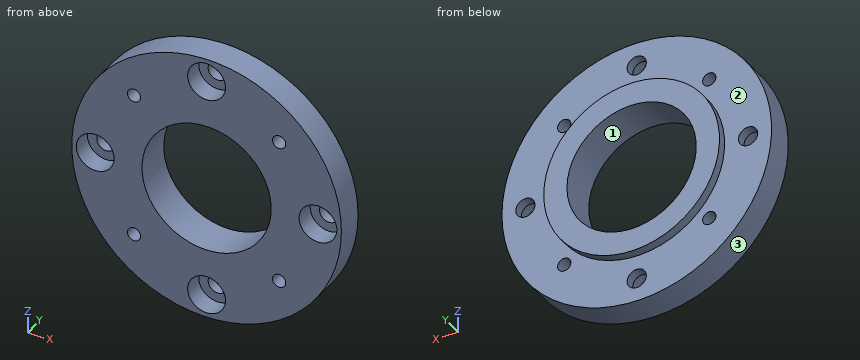
from build123d import *

# Parameters (mm, degrees)
SKETCH2_R                                      = 22.985
SKETCH2_R_2                                    = 1.63
SKETCH2_R_3                                    = 1.13
SKETCH2_R_4                                    = 14.985
SKETCH2_R_5                                    = 11.025
BOSS_EXTRUDE1_DEPTH                            = 4.95
BOSS_EXTRUDE2_START                            = 4.95
SKETCH2_3_R                                    = 14.985
SKETCH2_3_R_2                                  = 11.025
BOSS_EXTRUDE2_DEPTH                            = 1.52
F_4_40_TAPPED_HOLE1_D                          = 2.2606
CBORE_FOR_4_SOCKET_HEAD_CAP_SCREW1_D           = 3.2639
CBORE_FOR_4_SOCKET_HEAD_CAP_SCREW1_CBORE_D     = 6.450000054
CBORE_FOR_4_SOCKET_HEAD_CAP_SCREW1_CBORE_DEPTH = 3.300000004


with BuildPart() as part:
    # Sketch2 → Boss-Extrude1 (new body)
    with BuildSketch(Plane(origin=(0, 0, 0), x_dir=(1, 0, 0), z_dir=(0, 1, 0))):
        Circle(SKETCH2_R)
        with Locations((-18.99, 0)):
            Circle(SKETCH2_R_2, mode=Mode.SUBTRACT)
        with Locations((0, -18.99)):
            Circle(SKETCH2_R_2, mode=Mode.SUBTRACT)
        with Locations((18.99, 0)):
            Circle(SKETCH2_R_2, mode=Mode.SUBTRACT)
        with Locations((0, 18.99)):
            Circle(SKETCH2_R_2, mode=Mode.SUBTRACT)
        with Locations((12.367297603, -12.367297603)):
            Circle(SKETCH2_R_3, mode=Mode.SUBTRACT)
        with Locations((-12.367297603, -12.367297603)):
            Circle(SKETCH2_R_3, mode=Mode.SUBTRACT)
        with Locations((12.367297603, 12.367297603)):
            Circle(SKETCH2_R_3, mode=Mode.SUBTRACT)
        with Locations((-12.367297603, 12.367297603)):
            Circle(SKETCH2_R_3, mode=Mode.SUBTRACT)
        Circle(SKETCH2_R_4, mode=Mode.SUBTRACT)
        Circle(SKETCH2_R_4)
        Circle(SKETCH2_R_5, mode=Mode.SUBTRACT)
    extrude(amount=BOSS_EXTRUDE1_DEPTH)

    # Sketch2<3> → Boss-Extrude2 (add)
    with BuildSketch(Plane(origin=(0, 0, 0), x_dir=(1, 0, 0), z_dir=(0, 1, 0)).offset(BOSS_EXTRUDE2_START)):
        Circle(SKETCH2_3_R)
        Circle(SKETCH2_3_R_2, mode=Mode.SUBTRACT)
    extrude(amount=BOSS_EXTRUDE2_DEPTH)

    # #4-40 Tapped Hole1 (through all)
    with Locations(Plane(origin=(12.367297603, 4.95, -12.367297603), x_dir=(0, 0, 1), z_dir=(0, 1, 0))):
        with Locations((0, 0), (24.734595206, 0), (24.734595206, -24.734595206), (0, -24.734595206)):
            Hole(F_4_40_TAPPED_HOLE1_D / 2)

    # CBORE for #4 Socket Head Cap Screw1 (through all)
    with Locations(Plane(origin=(0, 0, 18.99), x_dir=(0, 0, -1), z_dir=(0, -1, 0))):
        with Locations((0, 0), (18.99, 18.99), (37.98, 0), (18.99, -18.99)):
            CounterBoreHole(CBORE_FOR_4_SOCKET_HEAD_CAP_SCREW1_D / 2, CBORE_FOR_4_SOCKET_HEAD_CAP_SCREW1_CBORE_D / 2, CBORE_FOR_4_SOCKET_HEAD_CAP_SCREW1_CBORE_DEPTH)


solid = part.part
The model under review builds one solid part; all positions refer to its coordinate system, in mm. Face numbers are marked on the shaded views. Round coordinates to 2 decimals unless told otherwise and drop trailing zeros. Write each loop counter-clockwise with the first axis right and the second up, starting at its lowest first coordinate (ties: lowest second). Pieces come first, ordered by that corner, then holes. Notation, with made-up numbers: (22, 6.25) - (62, 6.25) arc R25 cw to (62, 25.25) - close; hole circle Ø11 at (15.5, 29). An arc over 180 degrees is marked (long way). One line per item, written item: value. Start each with the question number.
1. Consider section A-A on z = 8. Write out the cut boundary in (x, y).
2. Clearance check with flat-ended pins moving along their axes: P1, Ø4, axis at x = 0, z = -18.99, coming from the -Y side; P2, Ø17.5, axis at x = 0, z = 0, coming from the -Y side; P3, Ø2.5, axis at x = -12.37, z = -12.37, coming from the +Y side; P4, Ø2, axis at x = -17, y = 5, coming from the -Z side. State where each tip first meets the part, or that it passes through.
3. Consider section C-C on x = 18.99. Write out the cut boundary in (y, z) (3 decimals).
4. Consider section B-B on x = 1. Write out the cut boundary in (y, z).
5. The part is to be moulded in two halves that separate along Z. For the marked faces 1, 2 and 3, say which applies: released by +Z, released by -Z, zero draft, split by the parting line, or undercut.
6. To check wall thickness, follow L1, parallel to X at y = 3.95, z = 0 (3 decimals); L2, parallel to X at y = 2, z = 0 (3 decimals); L3, parallel to Z at x = 11.5, y = 1.75. State the ranges of each line that lie inside material, in increasing order. Write a range as from..to.
Checks:
1. outline: (-21.55, 0) - (-7.59, 0) - (-7.59, 6.47) - (-12.67, 6.47) - (-12.67, 4.95) - (-21.55, 4.95) - close; (7.59, 0) - (21.55, 0) - (21.55, 4.95) - (12.67, 4.95) - (12.67, 6.47) - (7.59, 6.47) - close
2. P1: stops at y = 3.3
2. P2: passes through
2. P3: stops at y = 4.95
2. P4: stops at z = -16.5
3. outline: (0, -12.95) - (4.95, -12.95) - (4.95, -1.632) - (3.3, -1.632) - (3.3, -3.225) - (0, -3.225) - close; (0, 3.225) - (3.3, 3.225) - (3.3, 1.632) - (4.95, 1.632) - (4.95, 12.95) - (0, 12.95) - close
4. outline: (0, -22.96) - (4.95, -22.96) - (4.95, -20.28) - (3.3, -20.28) - (3.3, -22.06) - (0, -22.06) - close; (0, -15.92) - (3.3, -15.92) - (3.3, -17.7) - (4.95, -17.7) - (4.95, -14.95) - (6.47, -14.95) - (6.47, -10.98) - (0, -10.98) - close; (0, 10.98) - (6.47, 10.98) - (6.47, 14.95) - (4.95, 14.95) - (4.95, 17.7) - (3.3, 17.7) - (3.3, 15.92) - (0, 15.92) - close; (0, 22.06) - (3.3, 22.06) - (3.3, 20.28) - (4.95, 20.28) - (4.95, 22.96) - (0, 22.96) - close
5. face 1: undercut
5. face 2: zero draft
5. face 3: split by the parting line
6. L1: x = -22.985..-20.622, -17.358..-11.025, 11.025..17.358, 20.622..22.985
6. L2: x = -22.985..-22.215, -15.765..-11.025, 11.025..15.765, 22.215..22.985
6. L3: z = -19.9..-13.09, -11.64..11.64, 13.09..19.9
